Build history of the part. All positions in model axes, mm. A direction names the side the tool comes from. Round coordinates to 2 decimals unless told otherwise and drop trailing zeros. Write each loop counter-clockwise with the first axis right and the second up, starting at its lowest first coordinate (ties: lowest second). Pieces come first, ordered by that corner, then holes.
1) Which spindle directions (+Z, -Z, +X, -X, +Y, -Y) get a long thin tool onto all of the face, cutting with end or side? Do faces 1 (the flat face through (23, 3, 10)), 2 (the flat face through (0, 2, 109)). Say none if no direction does.
2) Saw through at A-A (z = 88.5). Write the cut outline in (x, y) (3 decimals).
3) Flat gauge pins, fed straight in: pin 1 (1.2 mm diameter, centred on y = 3, z = 214.5, fed in from +X); pin 2 (1 mm diameter, centred on y = 0.5, z = 146, fed in from +X); pin 3 (3 mm diameter, centred on x = 196, y = 2.5, fed in from -Z); pin 4 (2 mm diameter, centred on x = 118, z = 124.5, fed in from -Y). Where does each tip first touch, or does it go through?
4) Saw through at C-C (y = 2.2). Write the cut outline in (x, z).
5) Saw through at B-B (x = 164). Write the cut outline in (y, z), plus the area to 3 significant figures.
6) Wall check: probe 1 along Y at (x, z) = (47, 101); probe 2 along Z at (x, y) = (107.5, 1.85); probe 3 along Y at (x, z) = (53, 147). Give the ranges that are in metal, low to high.
Autodesk Inventor part; units mm, degrees
ref_plane "YZ Plane" through (0, 0, 0) normal (1, 0, 0) x (0, 1, 0)
ref_plane "XZ Plane" through (0, 0, 0) normal (0, 1, 0) x (-1, 0, 0)
ref_plane "XY Plane" through (0, 0, 0) normal (0, 0, 1) x (1, 0, 0)
sketch "スケッチ1" plane through (0, 0, 0) normal (0, 1, 0) x (-1, 0, 0)
  point P0 (0, 0)
sketch "スケッチ2" plane through (0, 0, 0) normal (0, 0, 1) x (1, 0, 0)
  line L0 (0, 0) -> (0, 5)
  line L1 (0, 5) -> (210, 1)
  line L2 (0, 0) -> (210, 0)
  line L3 (210, 1) -> (210, 0)
  dimension "d0" = 5
  dimension "d1" = 210
  dimension "d28" = 1
extrude "押し出し1" add sketch "スケッチ2" along normal blind 220
sketch "スケッチ4" plane through (0, 0, 220) normal (0, 0, 1) x (1, 0, 0)
  line L0 (0, 5) -> (0, 0)
  line L1 (55, 0) -> (245, 0)
  line L2 (245, 0) -> (245, 5)
  line L3 (245, 5) -> (55, 5)
  line L4 (55, 5) -> (55, 0)
  line L5 (0, 5) -> (45, 5)
  line L6 (45, 5) -> (45, 0)
  line L7 (45, 0) -> (0, 0)
  line L8 (0, 0) -> (0, 5)
  point P0 (0, 0)
  dimension "d8" = 5
  dimension "d9" = 190
  dimension "d10" = 55
  dimension "d23" = 45
  dimension "d30" = 5
extrude "押し出し2" cut sketch "スケッチ4" against normal blind 10
sketch "スケッチ5" plane through (0, 0, 0) normal (0, 0, -1) x (-1, 0, 0)
  line L0 (-55, 0) -> (-245, 0)
  line L1 (-245, 0) -> (-245, 4)
  line L2 (-245, 4) -> (-55, 4)
  line L3 (-55, 4) -> (-55, 0)
  line L4 (0, 5) -> (0, 0)
  line L5 (0, 5) -> (-45, 5)
  line L6 (-45, 5) -> (-45, 0)
  line L7 (-45, 0) -> (0, 0)
  line L8 (0, 0) -> (0, 5)
  dimension "d13" = 4
  dimension "d14" = 55
  dimension "d15" = 190
  dimension "d22" = 45
  dimension "d29" = 5
extrude "押し出し3" cut sketch "スケッチ5" against normal blind 10
sketch "スケッチ7" plane through (0, 0, 10) normal (-1, 0, 0) x (0, 0, 1)
  line L0 (200, 0) -> (200, 5)
  line L1 (200, 5) -> (0, 1)
  line L2 (0, 0) -> (200, 0)
  line L3 (0, 1) -> (0, 0)
  point P0 (-10, 0)
  dimension "d24" = 5
  dimension "d27" = 200
  dimension "d31" = 1
extrude "押し出し5" add sketch "スケッチ7" against normal blind 245
sketch "スケッチ6" plane through (0, 0, 0) normal (0, -1, 0) x (1, 0, 0)
  line L0 (0, 0) -> (0, 220)
  line L1 (55, 10) -> (210, 10)
  line L2 (245, 23.5) -> (146, 210)
  line L3 (245, 210) -> (245, 23.5)
  line L4 (146, 210) -> (245, 23.5)
  line L5 (146, 210) -> (245, 210)
  line L6 (210, 210) -> (55, 210)
  point P0 (235, 210)
  point P1 (235, 10)
  dimension "d18" = 146
  dimension "d19" = 13.5
extrude "押し出し4" cut sketch "スケッチ6" against normal blind 10
properties part number "坂"
Evaluation:
1. face 1: -Z, -X, +Y, -Y
1. face 2: +Z, -Z, -X, +Y, -Y
2. outline: (0, 0) - (210.496, 0) - (210.496, 2.57) - (127.575, 2.57) - (0, 5) - close
3. pin 1: stops at x = 55
3. pin 2: stops at x = 180.24
3. pin 3: stops at z = 10
3. pin 4: stops at y = 0
4. outline: (0, 10) - (45, 10) - (45, 0) - (55, 0) - (55, 10) - (147, 10) - (147, 70) - (220.32, 70) - (146, 210) - (55, 210) - (55, 220) - (45, 220) - (45, 210) - (0, 210) - close
5. outline: (0, 10) - (1.88, 10) - (1.88, 53.81) - (4.32, 176.09) - (0, 176.09) - close
5. area: 461 mm2
6. probe 1: y = 0 to 4.1
6. probe 2: z = 10 to 210
6. probe 3: y = 0 to 3.99
